```python
from build123d import *

# Parameters (mm, degrees)
F0_W     = 76.5
F0_H     = 55
F0_R     = 5
F1_DEPTH = 6.3


with BuildPart() as f1:
    # F0 (on Top) → F1 (new body)
    with BuildSketch(Plane.XY):
        Rectangle(F0_W, F0_H)
        with BuildLine():
            ThreePointArc((10.248019, 2.999999), (12.37062, 2.12202), (13.25, 0))
            ThreePointArc((13.25, 0), (12.371037, -2.121604), (10.249198, -3))
            Line((10.249198, -3), (-24.015752, -2.990841))
            ThreePointArc((-24.015752, -2.990841), (-24.250802, -3), (-24.485847, -2.990715))
            ThreePointArc((-24.485847, -2.990715), (-27.249231, -0.067905), (-24.620961, 2.976976))
            ThreePointArc((-24.620961, 2.976976), (-24.251981, 2.999999), (-23.882971, 2.977464))
            Line((-23.882971, 2.977464), (10.248019, 2.999999))
        make_face(mode=Mode.SUBTRACT)
        with Locations((25.25, 0)):
            Circle(F0_R, mode=Mode.SUBTRACT)
    extrude(amount=F1_DEPTH)


solid = f1.part
```
Input: part model. Units: mm. Frame: model coordinates. Round coordinates to 2 decimals unless told otherwise and drop trailing zeros. Loops run counter-clockwise (first coordinate to the right, second up) from the corner with the lowest first, then second, coordinate; pieces in that order, holes last. Notation, with made-up numbers: (-8, 84) - (38, 84) arc R19 ccw to (38, 100) - close; hole circle Ø5 at (66.5, 13.25). An arc over 180 degrees is marked (long way). One line per item, written item: value. Start each with the question number.
(1) Section C-C, the plane x = -6.5. Return loops of the section in (y, z), plus the area to 3 significant figures.
(2) Ray query, line 1 (Y direction, x = -17.5, z = 4.5); line 2 (Y direction, x = 25.25, z = 2.5). Return the intervals inside material, ascending. Write a range as [from, to].
(3) Section B-B, the plane z = 3.25. Return loops of the section in (x, y).
(4) Draft query along X for faces 1 (the cylindrical face through (-27.247, -0.13, 3.106)), 2 (the flat face through (-38.25, 0, 3)), 3 (the flat face through (-1, 27.5, 3)). Return one class per face: +X half, -X half, draft (parallel to the pull), parting line (faces both ways), or undercut.
(5) Section A-A, the plane x = 25.25. Return loops of the section in (y, z), plus the area to 4 significant figures.
Results below:
1. outline: (-27.5, 0) - (-3, 0) - (-3, 6.3) - (-27.5, 6.3) - close; (2.99, 0) - (27.5, 0) - (27.5, 6.3) - (2.99, 6.3) - close
1. area: 309 mm^2
2. line 1: [-27.5, -2.99], [2.98, 27.5]
2. line 2: [-27.5, -5], [5, 27.5]
3. outline: (-38.25, -27.5) - (38.25, -27.5) - (38.25, 27.5) - (-38.25, 27.5) - close; hole (-24.62, 2.98) arc R3 ccw to (-24.49, -2.99) arc R3 ccw to (-24.02, -2.99) - (10.25, -3) arc R3 ccw to (10.25, 3) - (-23.88, 2.98) arc R3 ccw to start; hole circle Ø10 at (25.25, 0)
4. face 1: undercut
4. face 2: -X half
4. face 3: draft
5. outline: (-27.5, 0) - (-5, 0) - (-5, 6.3) - (-27.5, 6.3) - close; (5, 0) - (27.5, 0) - (27.5, 6.3) - (5, 6.3) - close
5. area: 283.5 mm^2
